Can you work these out from the model? Positions are in its coordinate system, mm. Face numbers are marked on the shaded views. A direction names the side the tool comes from. Round coordinates to 2 decimals unless told otherwise and drop trailing zeros. Write each loop counter-clockwise with the first axis right and the second up, starting at its lowest first coordinate (ties: lowest second). Pieces come first, ordered by that corner, then holes.
Q1. If we section it at C-C (x = 7.5): Please give me the cut outline in (y, z) (1 decimal), plus the area to 3 significant figures.
Q2. I'm going to push flat-ended pins straight in: pin 1 Ø6.5 at (x, y) = (1, -1.5) entering from +Z; pin 2 Ø1 at (x, z) = (-1.5, -1.5) entering from +Y; pin 3 Ø1.6 at (y, z) = (1, -2) entering from -X; pin 4 Ø2.5 at (x, y) = (0, 0) entering from -Z. Where does each tip first touch, or does it pass through?
Q3. If we section it at D-D (z = -3): Please give me the cut outline in (x, y) (3 decimals), plus the area to 3 significant figures.
Q4. If we section it at B-B (y = 0): Please give me the cut outline in (x, z).
Q5. Please list where these lines run through material, in increasing order: line 1 along Y through (x, z) = (0, 0.45); line 2 along Y through (x, z) = (8.5, -2.5) (3 decimals); line 3 along Y through (x, z) = (6.5, -1.25).
Q6. For the marked faces 4, 5, 6, 7 and 8, which set-ups out of +Z, -Z, +X, -X, +Y, -Y let a thin tool reach every point of the face, with its end or its side?
Q7. We'd pull the mould along Y, two halves only. Please class the marked faces 1, 2 and 3: +Y half, -Y half, draft (parallel to the pull), parting line (faces both ways), or undercut.
Q8. If we section it at A-A (z = 2.75): Please give me the cut outline in (x, y) (3 decimals), plus the area to 3 significant figures.
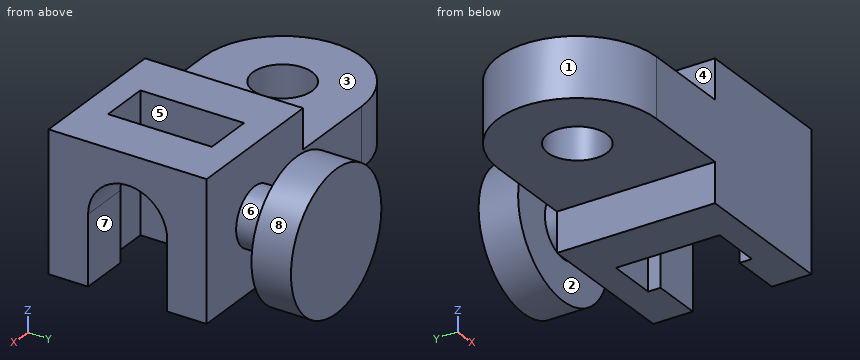
from build123d import *

# Parameters (mm, degrees)
SKETCH1_R               = 1.5
BOSS_EXTRUDE1_DEPTH     = 1.5
SKETCH5_W               = 7.463090523
SKETCH5_H               = 8
BOSS_EXTRUDE2_DEPTH     = 3.5
CUT_EXTRUDE1_DEPTH      = 7
CUT_EXTRUDE1_DEPTH_BACK = 6
SKETCH2_W               = 2.5
SKETCH2_H               = 5.25
SKETCH3_R               = 2
CUT_EXTRUDE2_DEPTH      = 3
SKETCH6_W               = 5
SKETCH6_H               = 4
CUT_EXTRUDE3_DEPTH      = 3.5
SKETCH7_R               = 1.45
BOSS_EXTRUDE3_DEPTH     = 2.1
SKETCH8_R               = 3.5
BOSS_EXTRUDE4_DEPTH     = 2


with BuildPart() as part:
    # Sketch1 → Boss-Extrude1 (new, symmetric)
    with BuildSketch(Plane.XY):
        with BuildLine():
            Line((12, 4), (0, 4))
            ThreePointArc((0, 4), (-4, 0), (0, -4))
            Line((0, -4), (12, -4))
            Line((12, -4), (12, 4))
        make_face()
        Circle(SKETCH1_R, mode=Mode.SUBTRACT)
    extrude(amount=BOSS_EXTRUDE1_DEPTH, both=True)

    # Sketch5 → Boss-Extrude2 (add, symmetric)
    with BuildSketch(Plane.XY):
        with Locations((8.268454739, 0)):
            Rectangle(SKETCH5_W, SKETCH5_H)
    extrude(amount=BOSS_EXTRUDE2_DEPTH, both=True)

    # Sketch2 → Cut-Extrude1 (cut, two sides: drawn at the far end of the back side and taken through both)
    with BuildSketch(Plane.XY.offset(1.5).offset(-CUT_EXTRUDE1_DEPTH_BACK)):
        with Locations((8.25, 0)):
            Rectangle(SKETCH2_W, SKETCH2_H)
    extrude(amount=CUT_EXTRUDE1_DEPTH + CUT_EXTRUDE1_DEPTH_BACK, mode=Mode.SUBTRACT)

    # Sketch3 → Cut-Extrude2 (cut)
    with BuildSketch(Plane(origin=(12, 0, 0), x_dir=(0, 0, -1), z_dir=(1, 0, 0))):
        with Locations(Location((0, 0, 0), (0, 0, 90))):
            Circle(SKETCH3_R)
    extrude(amount=-CUT_EXTRUDE2_DEPTH, mode=Mode.SUBTRACT)

    # Sketch6 → Cut-Extrude3 (cut)
    with BuildSketch(Plane(origin=(0, 0, -3.5), x_dir=(-1, 0, 0), z_dir=(0, 0, -1))):
        with Locations((-12, 0)):
            Rectangle(SKETCH6_W, SKETCH6_H)
    extrude(amount=-CUT_EXTRUDE3_DEPTH, mode=Mode.SUBTRACT)

    # Sketch7 → Boss-Extrude3 (add)
    with BuildSketch(Plane(origin=(0, 4, 0), x_dir=(1, 0, 0), z_dir=(0, 1, 0))):
        with Locations(Location((8.268454739, 0, 0), (0, 0, 180))):
            Circle(SKETCH7_R)
    extrude(amount=BOSS_EXTRUDE3_DEPTH)

    # Sketch8 → Boss-Extrude4 (add)
    with BuildSketch(Plane(origin=(0, 6.1, 0), x_dir=(1, 0, 0), z_dir=(0, 1, 0))):
        with Locations(Location((8.246364187, 0, 0), (0, 0, 180))):
            Circle(SKETCH8_R)
    extrude(amount=BOSS_EXTRUDE4_DEPTH)


solid = part.part
A:
1. outline: (-4, -3.5) - (-2.6, -3.5) - (-2.6, 3.5) - (-4, 3.5) - close; (2.6, -3.5) - (4, -3.5) - (4, -1.2) - (6.1, -1.2) - (6.1, -3.4) - (8.1, -3.4) - (8.1, 3.4) - (6.1, 3.4) - (6.1, 1.2) - (4, 1.2) - (4, 3.5) - (2.6, 3.5) - close
1. area: 38.1 mm2
2. pin 1: stops at z = 1.5
2. pin 2: stops at y = 3.87
2. pin 3: stops at x = -3.98
2. pin 4: passes through
3. outline: (4.537, -4) - (12, -4) - (12, -2) - (9.5, -2) - (9.5, -2.625) - (7, -2.625) - (7, 2.625) - (9.5, 2.625) - (9.5, 2) - (12, 2) - (12, 4) - (4.537, 4) - close; (6.444, 6.1) - (10.049, 6.1) - (10.049, 8.1) - (6.444, 8.1) - close
3. area: 43.8 mm2
4. outline: (-4, -1.5) - (-1.5, -1.5) - (-1.5, 1.5) - (-4, 1.5) - close; (1.5, -1.5) - (4.54, -1.5) - (4.54, -3.5) - (7, -3.5) - (7, 3.5) - (4.54, 3.5) - (4.54, 1.5) - (1.5, 1.5) - close; (9.5, 2) - (12, 2) - (12, 3.5) - (9.5, 3.5) - close
5. line 1: y = -4 to -1.5, 1.5 to 4
5. line 2: y = -4 to -2.625, 2.625 to 4, 6.1 to 8.1
5. line 3: y = -4 to 4, 6.1 to 8.1
6. face 4: +Z, -X, +Y, -Y
6. face 5: +Z, -Z
6. face 6: none
6. face 7: -Z, +X
6. face 8: +Y
7. face 1: parting line
7. face 2: undercut
7. face 3: draft
8. outline: (4.537, -4) - (12, -4) - (12, 4) - (4.537, 4) - close; (6.081, 6.1) - (10.411, 6.1) - (10.411, 8.1) - (6.081, 8.1) - close; hole (7, -2.625) - (9.5, -2.625) - (9.5, 2.625) - (7, 2.625) - close
8. area: 55.2 mm2
